```python
from build123d import *

# Parameters (mm, degrees)
SKETCH1_R           = 8.595
BOSS_EXTRUDE1_DEPTH = 9.7
BOSS_EXTRUDE3_START = 1
SKETCH2_R           = 8.595
BOSS_EXTRUDE3_DEPTH = 1


with BuildPart() as part:
    # Sketch1 → Boss-Extrude1 (new body)
    with BuildSketch(Plane(origin=(0, 0, 0), x_dir=(1, 0, 0), z_dir=(0, 1, 0))):
        with Locations(Location((0, 0, 0), (0, 0, 270))):
            Circle(SKETCH1_R)
        with BuildLine():
            Line((2.921067116, 1.559875967), (-2.806515464, 1.559875967))
            ThreePointArc((-2.806515464, 1.559875967), (0.057275826, -3.308241049), (2.921067116, 1.559875967))
        make_face(mode=Mode.SUBTRACT)
    extrude(amount=BOSS_EXTRUDE1_DEPTH)

    # Sketch2 → Boss-Extrude3 (add)
    with BuildSketch(Plane.XZ.offset(BOSS_EXTRUDE3_START)):
        with Locations(Location((0, 0, 0), (0, 0, 270))):
            Circle(SKETCH2_R)
    extrude(amount=-BOSS_EXTRUDE3_DEPTH)


solid = part.part
```
Geometry check sheet. Reference: the model listing, model coordinates, mm. A direction names the side the tool comes from. Round coordinates to 2 decimals unless told otherwise and drop trailing zeros. Loops run counter-clockwise (first coordinate to the right, second up) from the corner with the lowest first, then second, coordinate; pieces in that order, holes last. Notation, with made-up numbers: (51.5, -34) - (57.5, -34) arc R16 cw to (57.5, -10) - close; hole circle Ø5 at (54.5, 79). An arc over 180 degrees is marked (long way). Write each question's results on one line, items separated by ' | '. Start each with the question number.
Q1. Cross-section at C-C on y = 0.5. Enter the section's corners in (x, z) (3 decimals), and give its area (3 significant figures).
Q2. Release check for a two-part mould opening along X. For faces 3 (the flat face through (0, 5, -1.56)), 4 (the flat face through (0, 9.7, -2)) record: +X half, -X half, draft (parallel to the pull), parting line (faces both ways), or undercut.
Q3. Cross-section at B-B on x = 0. Enter the section's corners in (y, z) (3 decimals), and give its area (3 significant figures).
Q4. Cross-section at A-A on z = -0.75. Enter the section's corners in (x, y), and give its area (3 significant figures).
Q5. Cross-section at D-D on x = 3.75. Enter the section's corners in (y, z).
Q6. Access from +Z, -Z, +X, -X, +Y, -Y to the whole of each face (thin tool, end or side, straight path). Record for faces 1 (the cylindrical face through (-0.038, 4.782, 3.307)), 2 (the flat face through (0, -1, 0)).
Q7. Thickness scan on line 1 (X direction, y = 3.5, z = -1.25); line 2 (X direction, y = 2, z = 1); line 3 (Y direction, x = 0.75, z = 3). Record the ranges inside material, lowest first. Write a range as [from, to].
Q8. Gauge pin test, flat ends, axial feed: P1, Ø5, axis at x = 4, y = 8, coming from the -Z side; P2, Ø3, axis at x = -2, y = 0.5, coming from the +Z side; P3, Ø2.5, axis at x = 0.5, z = 1.5, coming from the +Y side. Record the tip position at first contact, or that the pin passes through.
Answers below:
1) outline: circle Ø17.19 at (0, 0); hole (-2.807, -1.56) - (2.921, -1.56) arc R3.276 ccw (long way) to start | area: 205 mm²
2) face 3: undercut | face 4: draft
3) outline: (-1, -8.595) - (9.7, -8.595) - (9.7, -1.56) - (0, -1.56) - (0, 3.308) - (9.7, 3.308) - (9.7, 8.595) - (-1, 8.595) - close | area: 137 mm²
4) outline: (-8.56, -1) - (8.56, -1) - (8.56, 9.7) - (3.24, 9.7) - (3.24, 0) - (-3.12, 0) - (-3.12, 9.7) - (-8.56, 9.7) - close | area: 122 mm²
5) outline: (-1, -7.73) - (9.7, -7.73) - (9.7, 7.73) - (-1, 7.73) - close
6) face 1: +Y | face 2: +Z, -Z, +X, -X, -Y
7) line 1: x = [-8.5, -2.96], [3.07, 8.5] | line 2: x = [-8.54, -3.07], [3.19, 8.54] | line 3: y = [-1, 0]
8) P1: stops at z = -8.46 | P2: stops at z = 8.58 | P3: stops at y = 0
